Here's how the part is built. I have some questions about the finished solid (model axes, mm). A direction names the side the tool comes from. Coordinates: 2 decimals unless noted, no trailing zeros. Write each loop counter-clockwise with the first axis right and the second up, starting at its lowest first coordinate (ties: lowest second). Pieces come first, ordered by that corner, then holes. Notation, with made-up numbers: (69.5, -5.5) -> (121.5, -5.5) arc R5 ccw to (121.5, 3.5) -> close; hole circle Ø6 at (-36.75, 8.25). An arc over 180 degrees is marked (long way). Put each result on its own line as item: value.
```python
from build123d import *

# Parameters (mm, degrees)
BASPROSKE_W              = 8
BASPROSKE_H              = 6
TOOTHCUT_DEPTH           = 12.66190379
TEETHCUTS_COUNT          = 10
TEETHCUTS_ANGLE          = 324
BORSKE_R                 = 2.5
BORE_DEPTH               = 50.0000508
RESSALTO_EXTRUS_O3_DEPTH = 8


with BuildPart() as part:
    # BasProSke → Base-Revolve (revolve)
    with BuildSketch(Plane(origin=(0, 0, 0), x_dir=(1, 0, 0), z_dir=(0, 1, 0)), mode=Mode.PRIVATE) as base_revolve_sk:
        with Locations((4, 3)):
            Rectangle(BASPROSKE_W, BASPROSKE_H)
    revolve(base_revolve_sk.sketch.rotate(Axis((-10, 0, 0), (1, 0, 0)), 180), axis=Axis((-10, 0, 0), (1, 0, 0)))

    # TooCutSke → ToothCut (cut, through all)
    with BuildSketch(Plane(origin=(0, 0, 0), x_dir=(0, 0, -1), z_dir=(1, 0, 0))):
        with BuildLine():
            ThreePointArc((0.59278292, 3.701838653), (0, 3.749), (-0.59278292, 3.701838653))
            ThreePointArc((-0.59278292, 3.701838653), (-0.846593509, 4.924114224), (-1.775771316, 5.757784417))
            ThreePointArc((-1.775771316, 5.757784417), (0, 6.0254), (1.775771316, 5.757784417))
            ThreePointArc((1.775771316, 5.757784417), (0.846593509, 4.924114224), (0.59278292, 3.701838653))
        make_face()
    toothcut = extrude(amount=TOOTHCUT_DEPTH, mode=Mode.SUBTRACT)

    # TeethCuts: ToothCut ×10 about axis
    teethcuts_axis = Axis((-10, 0, 0), (1, 0, 0))
    for i in range(1, TEETHCUTS_COUNT):
        add(toothcut.rotate(teethcuts_axis, i * TEETHCUTS_ANGLE / (TEETHCUTS_COUNT - 1)), mode=Mode.SUBTRACT)

    # BorSke → Bore (cut, symmetric)
    with BuildSketch(Plane(origin=(0, 0, 0), x_dir=(0, 0, -1), z_dir=(1, 0, 0))):
        with Locations(Location((0, 0, 0), (0, 0, 180))):
            Circle(BORSKE_R)
    extrude(amount=BORE_DEPTH, both=True, mode=Mode.SUBTRACT)

    # Esboço1 → Ressalto-extrusão3 (add)
    with BuildSketch(Plane(origin=(8, 0, 0), x_dir=(0, 0, -1), z_dir=(1, 0, 0))):
        with BuildLine():
            ThreePointArc((2, 1.5), (0, 2.5), (-2, 1.5))
            Line((-2, 1.5), (2, 1.5))
        make_face()
        with BuildLine():
            Line((2, -1.5), (-2, -1.5))
            ThreePointArc((-2, -1.5), (0, -2.5), (2, -1.5))
        make_face()
    extrude(amount=-RESSALTO_EXTRUS_O3_DEPTH)


solid = part.part
```
Item 1: If we mould it in two halves opening along Y, with no side actions, what happens to faces 3 (the flat face through (0, 2, 0)), 4 (the cylindrical face through (3.94, 4.48, 2.21))? For each: released by +Y, released by -Y, zero draft, split by the parting line, or undercut.
Output:
face 3: zero draft
face 4: undercut
Item 2: Imagine slicing it at A-A on z = 0. Write out the boundary of the cut face in (x, y), then the cut area to 3 significant figures.
Output:
outline: (0, -3.75) -> (8, -3.75) -> (8, -1.5) -> (0, -1.5) -> close; (0, 1.5) -> (8, 1.5) -> (8, 3.75) -> (0, 3.75) -> close
area: 36.0 mm²
Item 3: Which directions (+Z, -Z, +X, -X, +Y, -Y) give clear straight access to the entire face, cutting with the end or side of a thin tool? Please do faces 1 (the flat face through (8, 2, 0)), 2 (the flat face through (4, 1.5, 0)).
Output:
face 1: +Z, -Z, +X, +Y, -Y
face 2: +X, -X
Item 4: Please list where these lines run through material, in increasing order: line 1 along Y through (x, z) = (4.25, 0); line 2 along Y through (x, z) = (3.25, 4); line 3 along Z through (x, y) = (1.5, 3.5). Write a range as from..to.
Output:
line 1: y = -3.75..-1.5, 1.5..3.75
line 2: y = -3.62..-1.97, -0.69..0.69, 1.97..3.62
line 3: z = -4.87..-3.61, -1.83..1.83, 3.61..4.87
Item 5: For P1, Ø2, axis at x = 1, y = 3.5, coming from the +Z side; P2, Ø2, axis at y = 0, z = -0.5, coming from the -X side; P3, Ø3, axis at x = 4.5, z = 0, coming from the +Y side; P4, Ø1.5, axis at x = 2.5, z = -0.5, coming from the -Y side, each with a flat end and sliding along its axis, tell me the tip position at first contact or that it passes through.
Output:
P1: stops at z = 4.92
P2: passes through
P3: stops at y = 5.61
P4: stops at y = -5.42
Item 6: Imagine slicing it at B-B on y = -4. Write out the boundary of the cut face in (x, z), then the cut area to 3 significant figures.
Output:
outline: (0, -2.1) -> (8, -2.1) -> (8, -0.58) -> (0, -0.58) -> close; (0, 0.58) -> (8, 0.58) -> (8, 2.1) -> (0, 2.1) -> close
area: 24.2 mm²
